Could you check a few things on this model? Use its own coordinates, in mm. A direction names the side the tool comes from. Coordinates: 2 decimals unless noted, no trailing zeros. Loops run counter-clockwise (first coordinate to the right, second up) from the corner with the lowest first, then second, coordinate; pieces in that order, holes last.
1) Thinking about a two-plate mould opening in X: for faces 6 (the face through (6.002, -7.412, 1.521)), 7 (the face through (8, -10, 0)), 8 (the face through (15.1, 0.86, -8.11)), 9 (the face through (0, 39, -7)), which applies, released by +X, released by -X, zero draft, split by the parting line, or undercut?
2) Imagine slicing it at C-C on z = -12. Please give me the cut outline in (x, y).
3) Imagine slicing it at D-D on x = 2. Please give me the cut outline in (y, z), plus the area to 3 significant figures.
4) Imagine slicing it at B-B on x = 8. Please give me the cut outline in (y, z).
5) Will these pins go through, and if not, where does the flat tip stop? P1, Ø5, axis at x = 7.5, z = -6, coming from the +Y side; P2, Ø8, axis at x = 9, z = -8.5, coming from the -Y side.
6) Imagine slicing it at A-A on y = -7.5. Please give me the cut outline in (x, z).
7) If I drill on line 1 along Y through (x, z) = (8, 1); line 2 along Y through (x, z) = (10.5, -14); line 3 along Z through (x, y) = (13.25, 63), over which ranges is the centre line in solid material (lowest first)?
8) For faces 1 (the face through (8, 0, -8)), 2 (the face through (15.1, 76.64, -8.11)), 3 (the face through (0.86, 76.6, -8.11)), 4 (the face through (0.86, -14.1, 1.52)), 5 (the face through (0.86, 0.9, -8.11)), which set-ups out of +Z, -Z, +X, -X, +Y, -Y let a thin tool reach every point of the face, with its end or its side?
```python
from build123d import *

# Parameters (mm, degrees)
SKETCH2_W           = 16
SKETCH2_H           = 77.5
BOSS_EXTRUDE1_DEPTH = 19
BOSS_EXTRUDE2_DEPTH = 3
SKETCH4_R           = 2
CUT_EXTRUDE1_DEPTH  = 23
FILLET1_R           = 3
FILLET2_R           = 3


with BuildPart() as part:
    # Sketch2 → Boss-Extrude1 (new body)
    with BuildSketch(Plane.XY):
        with Locations((8, 38.75)):
            Rectangle(SKETCH2_W, SKETCH2_H)
    extrude(amount=-BOSS_EXTRUDE1_DEPTH)

    # Sketch3 → Boss-Extrude2 (add)
    with BuildSketch(Plane.XY):
        Polygon((0, 77.5), (0, 92.5), (16, 92.5), (16, 0), (16, -15), (0, -15), align=None)
    extrude(amount=BOSS_EXTRUDE2_DEPTH)

    # Sketch4 → Cut-Extrude1 (cut, through all)
    with BuildSketch(Plane.XY.offset(3)):
        with Locations((8, 85)):
            Circle(SKETCH4_R)
        with Locations((8, -7.5)):
            Circle(SKETCH4_R)
    extrude(amount=-CUT_EXTRUDE1_DEPTH, mode=Mode.SUBTRACT)

    # Fillet1
    fillet1_edges = [part.edges().sort_by_distance(p)[0] for p in [
        (8, 77.5, -19),
        (0, 38.75, -19),
        (8, 0, -19),
        (16, 38.75, -19),
        (0, 0, -9.5),
        (0, 77.5, -9.5),
        (16, 77.5, -9.5),
        (16, 0, -9.5),
    ]]
    fillet(fillet1_edges, radius=FILLET1_R)

    # Fillet2
    fillet2_edges = [part.edges().sort_by_distance(p)[0] for p in [
        (0, -15, 1.5),
        (16, -15, 1.5),
        (16, 92.5, 1.5),
        (0, 92.5, 1.5),
    ]]
    fillet(fillet2_edges, radius=FILLET2_R)


solid = part.part
```
Filled in:
1. face 6: undercut
1. face 7: zero draft
1. face 8: released by +X
1. face 9: released by -X
2. outline: (0, 3) arc R3 ccw to (3, 0) - (13, 0) arc R3 ccw to (16, 3) - (16, 74.5) arc R3 ccw to (13, 77.5) - (3, 77.5) arc R3 ccw to (0, 74.5) - close
3. outline: (-14.83, 0) - (0.17, 0) - (0.17, -16) arc R2.83 ccw to (3, -18.83) - (74.5, -18.83) arc R2.83 ccw to (77.33, -16) - (77.33, 0) - (92.33, 0) - (92.33, 3) - (-14.83, 3) - close
3. area: 1,770 mm2
4. outline: (-15, 0) - (-9.5, 0) - (-9.5, 3) - (-15, 3) - close; (-5.5, 0) - (0, 0) - (0, -16) arc R3 ccw to (3, -19) - (74.5, -19) arc R3 ccw to (77.5, -16) - (77.5, 0) - (83, 0) - (83, 3) - (-5.5, 3) - close; (87, 0) - (92.5, 0) - (92.5, 3) - (87, 3) - close
5. P1: stops at y = 77.5
5. P2: stops at y = 0
6. outline: (0, 0) - (6, 0) - (6, 3) - (0, 3) - close; (10, 0) - (16, 0) - (16, 3) - (10, 3) - close
7. line 1: y = -15 to -9.5, -5.5 to 83, 87 to 92.5
7. line 2: y = 0 to 77.5
7. line 3: z = -18.99 to 3
8. face 1: -Z, +X, -X, -Y
8. face 2: -Z, +X, +Y
8. face 3: -Z, -X, +Y
8. face 4: +Z, -Z, -X, -Y
8. face 5: -Z, -X, -Y
